```python
from build123d import *

# Parameters (mm, degrees)
CUT_EXTRUDE1_DEPTH  = 406.4
BOSS_EXTRUDE2_DEPTH = 228.6


with BuildPart() as part:
    # Sketch1 → Revolve1 (revolve)
    with BuildSketch(Plane.XY):
        with BuildLine():
            Line((0, 0), (685.8, 0))
            Line((685.8, 0), (685.8, 63.5))
            Line((685.8, 63.5), (635, 63.5))
            Line((635, 63.5), (635, 65.405))
            add(Edge.make_bspline(
                [(0, 0), (0.002192115, 0.006290208), (0.007522969, 0.018367599), (0.022271668, 0.040384559), (0.056983677, 0.080426255), (0.109817079, 0.130424863), (0.181602896, 0.188889433), (0.283649616, 0.263361483), (0.406270252, 0.344359984), (0.550210431, 0.431764809), (0.715531562, 0.525146598), (0.956716029, 0.653660621), (1.331811412, 0.839140677), (1.970276917, 1.127501619), (3.115826799, 1.592189007), (5.163395415, 2.328403475), (8.933180628, 3.515485788), (16.022028295, 5.446250201), (28.261741777, 8.304992794), (49.178793555, 12.513579304), (77.957328785, 17.487301978), (112.870807325, 22.806136935), (151.857530338, 28.124197322), (190.903568879, 32.982699255), (229.995170685, 37.459233955), (269.123174714, 41.603760556), (308.282068326, 45.445401222), (347.467762428, 49.002567332), (386.677550901, 52.283613526), (425.909385738, 55.28952525), (465.161890457, 58.012752885), (504.434100625, 60.436186371), (538.814064528, 62.266460598), (568.294487813, 63.592457812), (591.989866174, 64.466582586), (607.876612197, 64.942044427), (620.867800744, 65.238425835), (628.943051519, 65.360798765), (632.980968041, 65.399904908), (635, 65.405)],
                knots=[0, 0, 0, 0, 0, 4.1322e-05, 8.2644e-05, 0.000165287, 0.000330575, 0.000495862, 0.00066115, 0.00095525, 0.001249349, 0.001548926, 0.001848503, 0.002664392, 0.003865965, 0.00592961, 0.009578293, 0.016270012, 0.028578882, 0.05187103, 0.088176104, 0.149698422, 0.211220737, 0.272743055, 0.334265373, 0.395787692, 0.457310011, 0.518832329, 0.580354648, 0.641876966, 0.703399285, 0.764921604, 0.826443922, 0.887966241, 0.9187274, 0.94948856, 0.97474428, 0.98737214, 1, 1, 1, 1, 1], degree=4))
        make_face()
    revolve(axis=Axis((0, 0, 0), (1, 0, 0)))

    # Sketch2 → Cut-Extrude1 (cut)
    with BuildSketch(Plane(origin=(685.8, 0, 0), x_dir=(0, 0, -1), z_dir=(1, 0, 0))):
        with BuildLine():
            Line((76.2, 19.05), (62.569253831, 19.05))
            ThreePointArc((62.569253831, 19.05), (64.692179094, 9.629952704), (65.405, 0))
            ThreePointArc((65.405, 0), (64.692179094, -9.629952704), (62.569253831, -19.05))
            Line((62.569253831, -19.05), (76.2, -19.05))
            Line((76.2, -19.05), (76.2, -18.415))
            Line((76.2, -18.415), (76.2, 18.415))
            Line((76.2, 18.415), (76.2, 19.05))
        make_face()
        with BuildLine():
            ThreePointArc((-60.57513929, -19.05), (-63.5, 0), (-60.57513929, 19.05))
            Line((-60.57513929, 19.05), (-62.569253831, 19.05))
            ThreePointArc((-62.569253831, 19.05), (-65.405, 0), (-62.569253831, -19.05))
            Line((-62.569253831, -19.05), (-60.57513929, -19.05))
        make_face()
        with BuildLine():
            Line((62.569253831, 19.05), (60.57513929, 19.05))
            ThreePointArc((60.57513929, 19.05), (62.764525589, 9.636613904), (63.5, 0))
            ThreePointArc((63.5, 0), (62.764525589, -9.636613904), (60.57513929, -19.05))
            Line((60.57513929, -19.05), (62.569253831, -19.05))
            ThreePointArc((62.569253831, -19.05), (64.692179094, -9.629952704), (65.405, 0))
            ThreePointArc((65.405, 0), (64.692179094, 9.629952704), (62.569253831, 19.05))
        make_face()
        with BuildLine():
            ThreePointArc((-62.569253831, -19.05), (-65.405, 0), (-62.569253831, 19.05))
            Line((-62.569253831, 19.05), (-76.2, 19.05))
            Line((-76.2, 19.05), (-76.2, 18.415))
            Line((-76.2, 18.415), (-76.2, -18.415))
            Line((-76.2, -18.415), (-76.2, -19.05))
            Line((-76.2, -19.05), (-62.569253831, -19.05))
        make_face()
        with BuildLine():
            ThreePointArc((-60.57513929, -19.05), (-63.5, 0), (-60.57513929, 19.05))
            Line((-60.57513929, 19.05), (-62.569253831, 19.05))
            ThreePointArc((-62.569253831, 19.05), (-65.405, 0), (-62.569253831, -19.05))
            Line((-62.569253831, -19.05), (-60.57513929, -19.05))
        make_face()
        with BuildLine():
            Line((62.569253831, 19.05), (60.57513929, 19.05))
            ThreePointArc((60.57513929, 19.05), (62.764525589, 9.636613904), (63.5, 0))
            ThreePointArc((63.5, 0), (62.764525589, -9.636613904), (60.57513929, -19.05))
            Line((60.57513929, -19.05), (62.569253831, -19.05))
            ThreePointArc((62.569253831, -19.05), (64.692179094, -9.629952704), (65.405, 0))
            ThreePointArc((65.405, 0), (64.692179094, 9.629952704), (62.569253831, 19.05))
        make_face()
        with BuildLine():
            Line((-38.1, -19.05), (-38.1, 19.05))
            Line((-38.1, 19.05), (-60.57513929, 19.05))
            ThreePointArc((-60.57513929, 19.05), (-63.5, 0), (-60.57513929, -19.05))
            Line((-60.57513929, -19.05), (-38.1, -19.05))
        make_face()
        with BuildLine():
            Line((60.57513929, 19.05), (38.1, 19.05))
            Line((38.1, 19.05), (38.1, -19.05))
            Line((38.1, -19.05), (60.57513929, -19.05))
            ThreePointArc((60.57513929, -19.05), (62.764525589, -9.636613904), (63.5, 0))
            ThreePointArc((63.5, 0), (62.764525589, 9.636613904), (60.57513929, 19.05))
        make_face()
    extrude(amount=-CUT_EXTRUDE1_DEPTH, mode=Mode.SUBTRACT)

    # Sketch5 → Boss-Extrude2 (add)
    with BuildSketch(Plane(origin=(685.8, 0, 0), x_dir=(0, 0, -1), z_dir=(1, 0, 0))):
        with BuildLine():
            Line((-60.57513929, 19.05), (-38.1, 19.05))
            Line((-38.1, 19.05), (-38.1, -19.05))
            Line((-38.1, -19.05), (-60.57513929, -19.05))
            ThreePointArc((-60.57513929, -19.05), (0, -63.5), (60.57513929, -19.05))
            Line((60.57513929, -19.05), (38.1, -19.05))
            Line((38.1, -19.05), (38.1, 19.05))
            Line((38.1, 19.05), (60.57513929, 19.05))
            ThreePointArc((60.57513929, 19.05), (0, 63.5), (-60.57513929, 19.05))
        make_face()
    extrude(amount=BOSS_EXTRUDE2_DEPTH)


solid = part.part
```
Can you work these out from the model? Positions are in its coordinate system, mm. A direction names the side the tool comes from. Coordinates: 2 decimals unless noted, no trailing zeros. Order: outer loops, then holes, each group sorted by start corner. A loop starts at its lowest first (then second) coordinate and runs counter-clockwise, first axis right, second up. Notation, with made-up numbers: (21.25, 54.5) - (60.25, 54.5) arc R34 ccw to (60.25, 87.5) - close; hole circle Ø3 at (-1, 71.25). An arc over 180 degrees is marked (long way). Answer in a Markdown table with one row per item.
1. If we mould it in two halves opening along Y, with no side actions, what happens to faces 4 (the flat face through (635, -64, 0)), 5 (the flat face through (663, 19.05, -47)), 6 (the cylindrical face through (772.74, -63.49, 1.13))? For each: pulls with the +Y half, pulls with the -Y half, needs draft (parallel to the pull), parting line crosses it, or undercut.
Reply:
| item | result |
|---|---|
| face 4 | needs draft |
| face 5 | undercut |
| face 6 | pulls with the -Y half |
2. For pin 1 (1.3 mm diameter, centred on y = -2, z = -40, fed in from +X); pin 2 (8 mm diameter, centred on y = 14.5, z = -46, fed in from +X); pin 3 (12 mm diameter, centred on x = 641.5, z = -55.5, fed in from -Y); pin 4 (4 mm diameter, centred on x = 686, z = -14.5, fed in from +Y), each with a flat end and sliding along its axis, tell me the tip position at first contact or that it passes through.
Reply:
| item | result |
|---|---|
| pin 1 | stops at x = 279.4 |
| pin 2 | passes through |
| pin 3 | stops at y = -39.77 |
| pin 4 | stops at y = 62.26 |
3. For faces 1 (the flat face through (592, 0, -38.1)), 2 (the flat face through (592, 0, 38.1)), 3 (the flat face through (635, 65, 0)), which set-ups out of +Z, -Z, +X, -X, +Y, -Y let a thin tool reach every point of the face, with its end or its side?
Reply:
| item | result |
|---|---|
| face 1 | -Z, +X |
| face 2 | +Z, +X |
| face 3 | +X, +Y |
4. If I drill on line 1 along Z through (x, y) = (377.5, 8); line 2 along Y through (x, z) = (673, 0); line 3 along Y through (x, z) = (824, 28.5), over which ranges is the centre line in solid material (lowest first)?
Reply:
| item | result |
|---|---|
| line 1 | z = -38.1 to 38.1 |
| line 2 | y = -63.5 to 63.5 |
| line 3 | y = -56.75 to 56.75 |
5. Suppose I cut it at A-A (x = 673.5). Please give me the cut outline in (y, z).
Reply:
| item | result |
|---|---|
| outline | (-19.05, -60.58) - (-19.05, -38.1) - (19.05, -38.1) - (19.05, -60.58) arc R63.5 ccw to (19.05, 60.58) - (19.05, 38.1) - (-19.05, 38.1) - (-19.05, 60.58) arc R63.5 ccw to start |
